For this review, take the finished solid that the model builds, in its own axes (mm). Face numbers are marked on the shaded views. A direction names the side the tool comes from. Give positions to 0.01 mm unless a question says otherwise; leave off trailing zeros. Loops run counter-clockwise (first coordinate to the right, second up) from the corner with the lowest first, then second, coordinate; pieces in that order, holes last. Notation, with made-up numbers: (67.25, 43) - (120.25, 43) arc R20 cw to (120.25, 74) - close; hole circle Ø2 at (34.5, 42). An arc over 180 degrees is marked (long way). Answer in a Markdown table with one row per item.
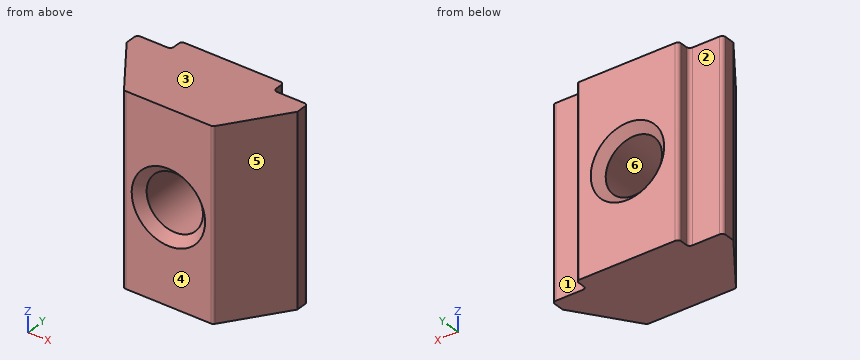
```python
from build123d import *

# Parameters (mm, degrees)
EXTRUDE_1_DEPTH = 5.5
FILLET_1_R      = 0.2


with BuildPart() as part:
    # Эскиз1 → Бобышка-Вытянуть1 (new body, symmetric)
    with BuildSketch(Plane.XY):
        Polygon((3, 0), (-3, 0), (-3, -0.8), (-5, -0.8), (-5, -1.6), (-2.6, -5), (2.6, -5), (5, -1.6), (5, -0.8), (3, -0.8), align=None)
    extrude(amount=EXTRUDE_1_DEPTH, both=True)

    # Эскиз4 → Отверстие обработанное метчиком M41 (revolve, cut)
    with BuildSketch(Plane(origin=(0, 0, 0), x_dir=(0, 0, 1), z_dir=(1, 0, 0))):
        Polygon((0, 0), (0, 5), (2.15, 5), (1.65, 4.5), (1.65, 0.5), (2.15, 0), align=None)
    revolve(axis=Axis((0, 6.35, 0), (0, -1, 0)), mode=Mode.SUBTRACT)

    # Скругление1
    fillet_1_edges = [part.edges().sort_by_distance(p)[0] for p in [
        (-3, 0, 0),
        (3, 0, 0),
        (3, -0.8, 0),
        (5, -0.8, 0),
        (2.6, -5, 0),
        (-2.6, -5, 0),
        (-5, -0.8, 0),
        (-3, -0.8, 0),
    ]]
    fillet(fillet_1_edges, radius=FILLET_1_R)


solid = part.part
```
1. Clearance check with flat-ended pins moving along their axes: pin 1 (0.8 mm diameter, centred on x = -4.5, z = -1, fed in from +Y); pin 2 (4 mm diameter, centred on x = 0, z = 0, fed in from +Y); pin 3 (5 mm diameter, centred on x = 4, z = 1.5, fed in from -Y). State where each tip first meets the part, or that it passes through.
Values:
| item | result |
|---|---|
| pin 1 | stops at y = -0.8 |
| pin 2 | stops at y = -0.15 |
| pin 3 | stops at y = -5 |
2. Mouldability with a two-part tool opening along X and no side actions: class the marked faces 4, 5 and 6 as released by +X, released by -X, zero draft, split by the parting line, or undercut.
Values:
| item | result |
|---|---|
| face 4 | zero draft |
| face 5 | released by +X |
| face 6 | undercut |
3. We need section B-B, the plane x = 0. Give the boundary of the cut face in (y, z), and give its area (3 significant figures).
Values:
| item | result |
|---|---|
| outline | (-5, -5.5) - (0, -5.5) - (0, -2.15) - (-0.5, -1.65) - (-4.5, -1.65) - (-5, -2.15) - close; (-5, 2.15) - (-4.5, 1.65) - (-0.5, 1.65) - (0, 2.15) - (0, 5.5) - (-5, 5.5) - close |
| area | 38.0 mm^2 |
4. We need section A-A, the plane z = 0. Give the boundary of the cut face in (x, y).
Values:
| item | result |
|---|---|
| outline | (-5, -1.6) - (-2.66, -4.92) arc R0.2 ccw to (-2.5, -5) - (-2.15, -5) - (-1.65, -4.5) - (-1.65, -0.5) - (-2.15, 0) - (-2.8, 0) arc R0.2 ccw to (-3, -0.2) - (-3, -0.6) arc R0.2 cw to (-3.2, -0.8) - (-4.8, -0.8) arc R0.2 ccw to (-5, -1) - close; (1.65, -4.5) - (2.15, -5) - (2.5, -5) arc R0.2 ccw to (2.66, -4.92) - (5, -1.6) - (5, -1) arc R0.2 ccw to (4.8, -0.8) - (3.2, -0.8) arc R0.2 cw to (3, -0.6) - (3, -0.2) arc R0.2 ccw to (2.8, 0) - (2.15, 0) - (1.65, -0.5) - close |
5. For the marked faces 1, 2 and 3, list the 3-axis set-ups (+Z, -Z, +X, -X, +Y, -Y) from which the entire face can be reached by the end or side of a thin tool; tool diameter is ignored.
Values:
| item | result |
|---|---|
| face 1 | +Z, -Z, +X, +Y |
| face 2 | +Z, -Z, -X, +Y |
| face 3 | +Z, +X, -X, +Y, -Y |
6. Wall thickness on line 1 (Z direction, x = 0, y = -2.2); line 2 (X direction, y = -2.15, z = 0.25); line 3 (X direction, y = -1.4, z = -1.5): over which ranges is each line inside the solid? List them lowest first. Write a range as [from, to].
Values:
| item | result |
|---|---|
| line 1 | z = [-5.5, -1.65], [1.65, 5.5] |
| line 2 | x = [-4.61, -1.63], [1.63, 4.61] |
| line 3 | x = [-5, -0.69], [0.69, 5] |
7. We need section D-D, the plane z = 4.25. Give the boundary of the cut face in (x, y).
Values:
| item | result |
|---|---|
| outline | (-5, -1.6) - (-2.66, -4.92) arc R0.2 ccw to (-2.5, -5) - (2.5, -5) arc R0.2 ccw to (2.66, -4.92) - (5, -1.6) - (5, -1) arc R0.2 ccw to (4.8, -0.8) - (3.2, -0.8) arc R0.2 cw to (3, -0.6) - (3, -0.2) arc R0.2 ccw to (2.8, 0) - (-2.8, 0) arc R0.2 ccw to (-3, -0.2) - (-3, -0.6) arc R0.2 cw to (-3.2, -0.8) - (-4.8, -0.8) arc R0.2 ccw to (-5, -1) - close |
8. We need section C-C, the plane y = -4.65. Give the boundary of the cut face in (x, z), and give its area (3 significant figures).
Values:
| item | result |
|---|---|
| outline | (-2.85, -5.5) - (2.85, -5.5) - (2.85, 5.5) - (-2.85, 5.5) - close; hole circle Ø3.6 at (0, 0) |
| area | 52.5 mm^2 |
